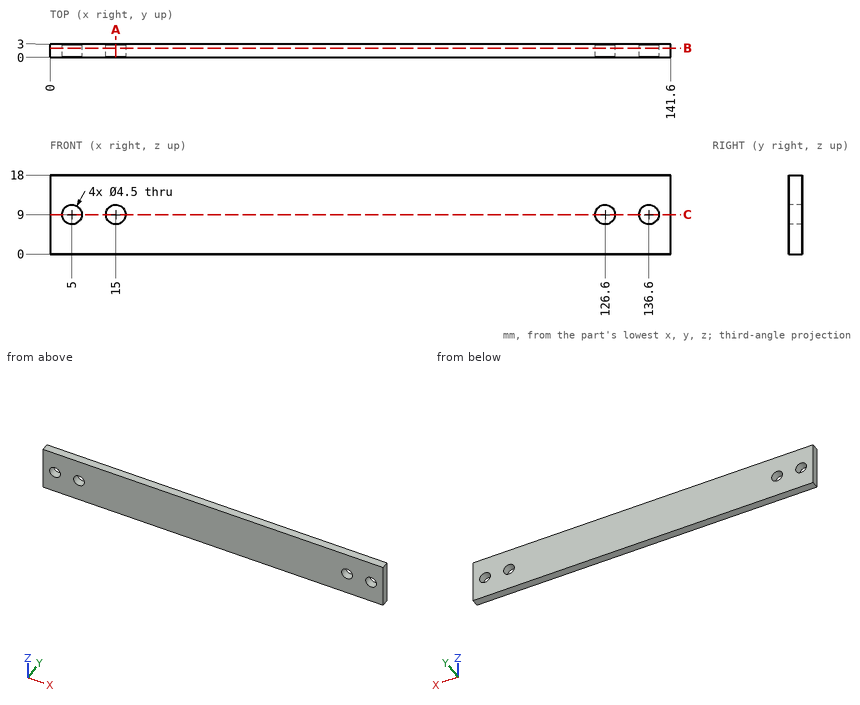
Design review of the part shown in the three views and the two pictorial views. Dimensions are in mm from the part's minimum x, y and z. Round coordinates to 2 decimals unless told otherwise and drop trailing zeros. Loops run counter-clockwise (first coordinate to the right, second up) from the corner with the lowest first, then second, coordinate; pieces in that order, holes last. Notation, with made-up numbers: (48, -20) -> (61, -20) arc R23 ccw to (61, 16) -> close; hole circle Ø4 at (24, -29.5). An arc over 180 degrees is marked (long way). Use one line per item in the form item = value. Start each with the question number.
Q1. We need section A-A on x = 15. Give the boundary of the cut face in (y, z), then the cut area to 3 significant figures.
Q2. We need section C-C on z = 9. Give the boundary of the cut face in (x, y), then the cut area to 3 significant figures.
Q3. For pin 1 Ø2 at (x, z) = (56.5, 11) entering from -Y; pin 2 Ø3.5 at (x, z) = (15, 9) entering from -Y, all flat-tipped, find the tip position at first contact; note any pin that passes through.
Q4. Wall thickness on line 1 along X through (y, z) = (1.9, 8.25); line 2 along Z through (x, y) = (126.6, 2.05); line 3 along X through (y, z) = (0.8, 8): over which ranges is each line inside the solid? List them lowest first. Write a range as [from, to].
Q5. We need section B-B on y = 2.05. Give the boundary of the cut face in (x, z).
Calculated:
q1.outline = (0, 0) -> (3, 0) -> (3, 6.75) -> (0, 6.75) -> close; (0, 11.25) -> (3, 11.25) -> (3, 18) -> (0, 18) -> close
q1.area = 40.5 mm²
q2.outline = (0, 0) -> (2.75, 0) -> (2.75, 3) -> (0, 3) -> close; (7.25, 0) -> (12.75, 0) -> (12.75, 3) -> (7.25, 3) -> close; (17.25, 0) -> (124.35, 0) -> (124.35, 3) -> (17.25, 3) -> close; (128.85, 0) -> (134.35, 0) -> (134.35, 3) -> (128.85, 3) -> close; (138.85, 0) -> (141.6, 0) -> (141.6, 3) -> (138.85, 3) -> close
q2.area = 371 mm²
q3.pin_1 = 0
q3.pin_2 = through
q4.line_1 = [0, 2.88], [7.12, 12.88], [17.12, 124.48], [128.72, 134.48], [138.72, 141.6]
q4.line_2 = [0, 6.75], [11.25, 18]
q4.line_3 = [0, 2.98], [7.02, 12.98], [17.02, 124.58], [128.62, 134.58], [138.62, 141.6]
q5.outline = (0, 0) -> (141.6, 0) -> (141.6, 18) -> (0, 18) -> close; hole circle Ø4.5 at (5, 9); hole circle Ø4.5 at (15, 9); hole circle Ø4.5 at (126.6, 9); hole circle Ø4.5 at (136.6, 9)
